from build123d import *

# Parameters (mm, degrees)
BOSS_EXTRUDE1_DEPTH     = 81
CUT_EXTRUDE1_DEPTH      = 42
CUT_EXTRUDE1_DEPTH_BACK = 42
SKETCH2_W               = 2931
SKETCH2_H               = 2169
SKETCH9_W               = 10
SKETCH9_H               = 10
CUT_EXTRUDE2_DEPTH      = 10
CUT_EXTRUDE3_START      = -28
SKETCH11_W              = 238.622036278
SKETCH11_H              = 213.304880218
SKETCH11_W_2            = 101.706666714
SKETCH11_H_2            = 70
CUT_EXTRUDE3_DEPTH      = 28
CHAMFER1_SIZE           = 0.4


with BuildPart() as part:
    # Sketch1 → Boss-Extrude1 (new body)
    with BuildSketch(Plane.XY):
        Polygon((-21, 12.5), (-21, 6), (-19.5, 3.401923789), (-19.5, -10), (-10, -10), (-6, -14), (6, -14), (10, -10), (19.5, -10), (19.5, 3.401923789), (21, 6), (21, 12.5), (19.5, 14), (8.75, 14), (8.35, 13.6), (-8.35, 13.6), (-8.75, 14), (-19.5, 14), align=None)
    extrude(amount=BOSS_EXTRUDE1_DEPTH)

    # Sketch2 → Cut-Extrude1 (cut, two sides: drawn at the far end of the back side and taken through both)
    with BuildSketch(Plane(origin=(0, 0, 0), x_dir=(0, 0, -1), z_dir=(1, 0, 0)).offset(-CUT_EXTRUDE1_DEPTH_BACK)):
        with Locations((-31.5, -9.5)):
            Rectangle(SKETCH2_W, SKETCH2_H)
        Polygon((-81, -14), (0, -14), (0, 13.6), (-0.4, 14), (-80.6, 14), (-81, 13.6), align=None, mode=Mode.SUBTRACT)
    extrude(amount=CUT_EXTRUDE1_DEPTH + CUT_EXTRUDE1_DEPTH_BACK, mode=Mode.SUBTRACT)

    # Sketch3 → Cut-Revolve1 (revolve, cut)
    with BuildSketch(Plane.XY.offset(15.5), mode=Mode.PRIVATE) as cut_revolve1_sk:
        Polygon((-15.25, 14), (-12.75, 14), (-13.183, 13.567), (-13.183, 2), (-13.1, 2), (-13.1, -10), (-15.25, -10), align=None)
    revolve(cut_revolve1_sk.sketch.rotate(Axis((-15.25, -10, 15.5), (0, 1, 0)), 270), axis=Axis((-15.25, -10, 15.5), (0, 1, 0)), mode=Mode.SUBTRACT)

    # Sketch4 → Cut-Revolve2 (revolve, cut)
    with BuildSketch(Plane.XY.offset(15.5), mode=Mode.PRIVATE) as cut_revolve2_sk:
        Polygon((15.25, 14), (17.75, 14), (17.317, 13.567), (17.317, 2), (17.4, 2), (17.4, -10), (15.25, -10), align=None)
    revolve(cut_revolve2_sk.sketch.rotate(Axis((15.25, -10, 15.5), (0, 1, 0)), 270), axis=Axis((15.25, -10, 15.5), (0, 1, 0)), mode=Mode.SUBTRACT)

    # Sketch5 → Cut-Revolve3 (revolve, cut)
    with BuildSketch(Plane.XY.offset(65.5), mode=Mode.PRIVATE) as cut_revolve3_sk:
        Polygon((-15.25, 14), (-12.75, 14), (-13.183, 13.567), (-13.183, 2), (-13.1, 2), (-13.1, -10), (-15.25, -10), align=None)
    revolve(cut_revolve3_sk.sketch.rotate(Axis((-15.25, -10, 65.5), (0, 1, 0)), 270), axis=Axis((-15.25, -10, 65.5), (0, 1, 0)), mode=Mode.SUBTRACT)

    # Sketch6 → Cut-Revolve4 (revolve, cut)
    with BuildSketch(Plane.XY.offset(65.5), mode=Mode.PRIVATE) as cut_revolve4_sk:
        Polygon((15.25, 14), (17.75, 14), (17.317, 13.567), (17.317, 2), (17.4, 2), (17.4, -10), (15.25, -10), align=None)
    revolve(cut_revolve4_sk.sketch.rotate(Axis((15.25, -10, 65.5), (0, 1, 0)), 270), axis=Axis((15.25, -10, 65.5), (0, 1, 0)), mode=Mode.SUBTRACT)

    # Sketch7 → Cut-Revolve5 (revolve, cut)
    with BuildSketch(Plane(origin=(0, 0, 0), x_dir=(0, 0, -1), z_dir=(1, 0, 0)), mode=Mode.PRIVATE) as cut_revolve5_sk:
        Polygon((-81, -1), (-81, 9.5), (-73.5, 9.5), (-73.5, 10), (-72.35, 10), (-72.35, 9.5), (-8.65, 9.5), (-8.65, 10), (-7.5, 10), (-7.5, 9.5), (0, 9.5), (0, -1), align=None)
    revolve(cut_revolve5_sk.sketch.rotate(Axis((0, -1, 0), (0, 0, 1)), 270), axis=Axis((0, -1, 0), (0, 0, 1)), mode=Mode.SUBTRACT)

    # Sketch8 → Revolve1 (revolve)
    with BuildSketch(Plane.XY.offset(40.5), mode=Mode.PRIVATE) as revolve1_sk:
        Polygon((19.5, 0), (19.5, 3.3), (20.5, 4.2), (21.5, 4.2), (24, 2.8), (25.3, 3.3), (28, 2.4), (28, 0), align=None)
    revolve(revolve1_sk.sketch.rotate(Axis((28, 0, 40.5), (-1, 0, 0)), 270), axis=Axis((28, 0, 40.5), (-1, 0, 0)))

    # Sketch9 → Cut-Extrude2 (cut)
    with BuildSketch(Plane(origin=(19.5, 0, 0), x_dir=(0, 0, -1), z_dir=(1, 0, 0))):
        with Locations((-40.5, 0)):
            Rectangle(SKETCH9_W, SKETCH9_H)
        Polygon((-44, 2.020725942), (-44, -2.020725942), (-40.5, -4.041451884), (-37, -2.020725942), (-37, 2.020725942), (-40.5, 4.041451884), align=None, mode=Mode.SUBTRACT)
    extrude(amount=CUT_EXTRUDE2_DEPTH, mode=Mode.SUBTRACT)

    # Sketch10 → Cut-Revolve6 (revolve, cut)
    with BuildSketch(Plane.XY.offset(40.5), mode=Mode.PRIVATE) as cut_revolve6_sk:
        Polygon((19.5, 4.2), (19.5, 3.3), (20.5, 4.2), align=None)
    revolve(cut_revolve6_sk.sketch.rotate(Axis((28, 0, 40.5), (-1, 0, 0)), 59.999999594), axis=Axis((28, 0, 40.5), (-1, 0, 0)), mode=Mode.SUBTRACT)

    # Sketch11 → Cut-Extrude3 (cut)
    with BuildSketch(Plane(origin=(0, 14, 0), x_dir=(1, 0, 0), z_dir=(0, 1, 0)).offset(CUT_EXTRUDE3_START)):
        with Locations((12.049646303, -40.5)):
            Rectangle(SKETCH11_W, SKETCH11_H)
        with Locations((12.049646303, -40.5)):
            Rectangle(SKETCH11_W_2, SKETCH11_H_2, mode=Mode.SUBTRACT)
    extrude(amount=CUT_EXTRUDE3_DEPTH, mode=Mode.SUBTRACT)

    # Chamfer1
    chamfer1_edges = [part.edges().sort_by_distance(p)[0] for p in [
        (-14.125, 14, 5.5),
        (14.125, 14, 5.5),
        (14.125, 14, 75.5),
        (-14.125, 14, 75.5),
    ]]
    chamfer(chamfer1_edges, length=CHAMFER1_SIZE)


solid = part.part
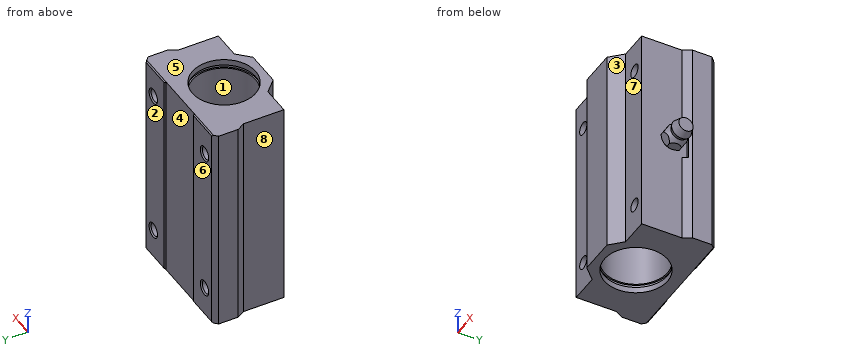
CAD build for the part. Positions are in the model's coordinates, mm. Face numbers are marked on the shaded views. A direction names the side the tool comes from. Coordinates: 2 decimals unless noted, no trailing zeros. Order: outer loops, then holes, each group sorted by start corner. A loop starts at its lowest first (then second) coordinate and runs counter-clockwise, first axis right, second up.
Item 1: Band-saw the part on D-D on z = 32. List the corners of the cut face in (x, y).
Check sheet entries:
outline: (-21, 6) - (-19.5, 3.4) - (-19.5, -10) - (-10, -10) - (-6, -14) - (6, -14) - (10, -10) - (19.5, -10) - (19.5, 3.4) - (21, 6) - (21, 12.5) - (19.5, 14) - (8.75, 14) - (8.35, 13.6) - (-8.35, 13.6) - (-8.75, 14) - (-19.5, 14) - (-21, 12.5) - close; hole circle Ø21 at (0, -1)
Item 2: Pin check, flat tips, straight feed: pin 1 Ø5 at (x, z) = (0.5, 64) entering from +Y; pin 2 Ø10.5 at (x, z) = (-14, 26) entering from -Y; pin 3 Ø6.5 at (y, z) = (-6.5, 32) entering from -X. Stop position of each tip, or through.
Check sheet entries:
pin 1: stops at y = 13.6
pin 2: stops at y = -11.25
pin 3: stops at x = -19.5
Item 3: Band-saw the part on B-B on z = 15.5. Give the number of separate pieces and of enclosed holes in the cut face, plus the area to 3 significant figures.
Check sheet entries:
separate pieces: 3
enclosed holes: 1
area: 470 mm2
Item 4: Band-saw the part on A-A on x = 15.25. List the corners of the cut face in (y, z), plus the area to 3 significant figures.
Check sheet entries:
outline: (-10, 5.5) - (13.6, 5.5) - (14, 5.9) - (14, 13) - (13.57, 13.43) - (2, 13.43) - (2, 13.35) - (-10, 13.35) - close; (-10, 17.65) - (2, 17.65) - (2, 17.57) - (13.57, 17.57) - (14, 18) - (14, 63) - (13.57, 63.43) - (2, 63.43) - (2, 63.35) - (-10, 63.35) - close; (-10, 67.65) - (2, 67.65) - (2, 67.57) - (13.57, 67.57) - (14, 68) - (14, 75.1) - (13.6, 75.5) - (-10, 75.5) - close
area: 1,480 mm2
Item 5: Drill centre lines: L1, parallel to Z at x = -15.5, y = -8.5; L2, parallel to X at y = -1, z = 5.9; L3, parallel to X at y = -2.75, z = 65.5. Where is each one in solid material? Low to high.
Check sheet entries:
L1: z = 5.5 to 13.36, 17.64 to 63.36, 67.64 to 75.5
L2: x = -19.5 to -10.5, 10.5 to 19.5
L3: x = -19.5 to -17.4, -13.1 to -10.35, 10.35 to 13.1, 17.4 to 19.5
Item 6: Two-plate mould, pull along X, no slides. Class the marked faces 1, 2 and 3: +X half, -X half, draft (parallel to the pull), parting line (faces both ways), or undercut.
Check sheet entries:
face 1: undercut
face 2: draft
face 3: +X half
Item 7: 3-axis set-ups, long thin cutter, end or side, ignore diameter. For the marked faces 4, 5, 6, 7 and 8: which of +Z, -Z, +X, -X, +Y, -Y reach the whole face in a straight line?
Check sheet entries:
face 4: +Z, -Z, +Y
face 5: +Z, +X, -X, +Y, -Y
face 6: +Z, -Z, +X, -X, +Y
face 7: +Z, -Z, +X, -Y
face 8: +Z, -Z, -X, -Y
Item 8: Band-saw the part on C-C on x = 0.5. List the corners of the cut face in (y, z), plus the area to 3 significant figures.
Check sheet entries:
outline: (-14, 5.5) - (-11.49, 5.5) - (-11.49, 7.5) - (-11.99, 7.5) - (-11.99, 8.65) - (-11.49, 8.65) - (-11.49, 72.35) - (-11.99, 72.35) - (-11.99, 73.5) - (-11.49, 73.5) - (-11.49, 75.5) - (-14, 75.5) - close; (9.49, 5.5) - (13.6, 5.5) - (13.6, 75.5) - (9.49, 75.5) - (9.49, 73.5) - (9.99, 73.5) - (9.99, 72.35) - (9.49, 72.35) - (9.49, 8.65) - (9.99, 8.65) - (9.99, 7.5) - (9.49, 7.5) - close
area: 461 mm2
